Geometry check sheet. Reference: the model listing, model coordinates, mm. A direction names the side the tool comes from. Give positions to 0.01 mm unless a question says otherwise; leave off trailing zeros. Order: outer loops, then holes, each group sorted by start corner. A loop starts at its lowest first (then second) coordinate and runs counter-clockwise, first axis right, second up.
```python
from build123d import *

# Parameters (mm, degrees)
SKETCH_W     = 42
SKETCH_H     = 42
PAD_DEPTH    = 48
CHAMFER_SIZE = 4
SKETCH005_R  = 18
PAD003_DEPTH = 35
SKETCH001_R  = 11
PAD001_DEPTH = 2
SKETCH002_R  = 4
PAD002_DEPTH = 20
POCKET_DEPTH = 15
SKETCH004_R  = 1.25
HOLE_DEPTH   = 4.5
HOLE_TIPS_R  = 1.25


with BuildPart() as part:
    # Sketch → Pad (new body)
    with BuildSketch(Plane.XY):
        Rectangle(SKETCH_W, SKETCH_H)
    extrude(amount=PAD_DEPTH)

    # Chamfer
    chamfer_edges = [part.edges().sort_by_distance(p)[0] for p in [
        (21, -21, 24),
        (-21, -21, 24),
        (21, 21, 24),
        (-21, 21, 24),
    ]]
    chamfer(chamfer_edges, length=CHAMFER_SIZE)

    # Sketch005 → Pad003 (join)
    with BuildSketch(Plane.XY):
        Circle(SKETCH005_R)
    extrude(amount=-PAD003_DEPTH)

    # Sketch001 → Pad001 (join)
    with BuildSketch(Plane.XY.offset(-35)):
        Circle(SKETCH001_R)
    extrude(amount=-PAD001_DEPTH)

    # Sketch002 (on Sketch) → Pad002 (join)
    with BuildSketch(Plane.XY.offset(-35)):
        Circle(SKETCH002_R)
    extrude(amount=-PAD002_DEPTH)

    # Sketch003 (on Sketch) → Pocket (cut)
    with BuildSketch(Plane.XY.offset(-40)):
        with BuildLine():
            ThreePointArc((10.583005, 3), (0, 11), (-10.583005, 3))
            Line((-10.583005, 3), (10.583005, 3))
        make_face()
    extrude(amount=-POCKET_DEPTH, mode=Mode.SUBTRACT)

    # Sketch004 (on Sketch) → Hole (cut)
    with BuildSketch(Plane.XY.offset(-35)):
        with Locations((9.899495, 9.899495)):
            Circle(SKETCH004_R)
        with Locations((-9.899495, 9.899495)):
            Circle(SKETCH004_R)
        with Locations((-9.899495, -9.899495)):
            Circle(SKETCH004_R)
        with Locations((9.899495, -9.899495)):
            Circle(SKETCH004_R)
    extrude(amount=HOLE_DEPTH, mode=Mode.SUBTRACT)

    # Hole tips → Hole tip 1 section 0
    with BuildSketch(Plane.XY.offset(-30.5), mode=Mode.PRIVATE) as hole_tip_1_s0:
        with Locations((9.899495, 9.899495)):
            Circle(HOLE_TIPS_R)
    loft([hole_tip_1_s0.sketch, Vertex(9.899495, 9.899495, -29.748924)], mode=Mode.SUBTRACT)

    # Hole tips → Hole tip 2 section 0
    with BuildSketch(Plane.XY.offset(-30.5), mode=Mode.PRIVATE) as hole_tip_2_s0:
        with Locations((-9.899495, 9.899495)):
            Circle(HOLE_TIPS_R)
    loft([hole_tip_2_s0.sketch, Vertex(-9.899495, 9.899495, -29.748924)], mode=Mode.SUBTRACT)

    # Hole tips → Hole tip 3 section 0
    with BuildSketch(Plane.XY.offset(-30.5), mode=Mode.PRIVATE) as hole_tip_3_s0:
        with Locations((-9.899495, -9.899495)):
            Circle(HOLE_TIPS_R)
    loft([hole_tip_3_s0.sketch, Vertex(-9.899495, -9.899495, -29.748924)], mode=Mode.SUBTRACT)

    # Hole tips → Hole tip 4 section 0
    with BuildSketch(Plane.XY.offset(-30.5), mode=Mode.PRIVATE) as hole_tip_4_s0:
        with Locations((9.899495, -9.899495)):
            Circle(HOLE_TIPS_R)
    loft([hole_tip_4_s0.sketch, Vertex(9.899495, -9.899495, -29.748924)], mode=Mode.SUBTRACT)


solid = part.part
```
Q1. Thickness scan on L1, parallel to Z at x = -2, y = 7.5; L2, parallel to Z at x = 14, y = -14; L3, parallel to X at y = 7, z = -0.5. Record the ranges inside material, lowest first.
Q2. Access from +Z, -Z, +X, -X, +Y, -Y to the whole of each face (thin tool, end or side, straight path). Record for faces 1 (the face through (21, 0, 24)), 2 (the face through (0, 3, -47)), 3 (the face through (-8, -8, -35)).
Q3. Cross-section at A-A, the plane z = 21. Record the boundary of the cut face in (x, y), and give its area (3 significant figures).
Q4. Gauge pin test, flat ends, axial feed: P1, Ø12.5, axis at x = 4.5, y = 9.5, coming from the -Z side; P2, Ø2, axis at y = 6.5, z = -31.5, coming from the +X side; P3, Ø0.8, axis at x = 0, y = 3.5, coming from the -Z side. Record the tip position at first contact, or that the pin passes through.
Q5. Cross-section at D-D, the plane y = 0. Record the boundary of the cut face in (x, z).
Q6. Cross-section at C-C, the plane y = -13. Record the boundary of the cut face in (x, z).
Q7. Cross-section at B-B, the plane x = 0. Record the boundary of the cut face in (y, z), and give its area (3 significant figures).
Answers follow:
1. L1: z = -37 to 48
1. L2: z = 0 to 48
1. L3: x = -16.58 to 16.58
2. face 1: +Z, -Z, +X, +Y, -Y
2. face 2: -Z, +X, -X, +Y
2. face 3: -Z
3. outline: (-21, -17) - (-17, -21) - (17, -21) - (21, -17) - (21, 17) - (17, 21) - (-17, 21) - (-21, 17) - close
3. area: 1,730 mm2
4. P1: stops at z = -37
4. P2: stops at x = 17.14
4. P3: stops at z = -40
5. outline: (-21, 0) - (-18, 0) - (-18, -35) - (-11, -35) - (-11, -37) - (-4, -37) - (-4, -55) - (4, -55) - (4, -37) - (11, -37) - (11, -35) - (18, -35) - (18, 0) - (21, 0) - (21, 48) - (-21, 48) - close
6. outline: (-21, 0) - (-12.45, 0) - (-12.45, -35) - (12.45, -35) - (12.45, 0) - (21, 0) - (21, 48) - (-21, 48) - close
7. outline: (-21, 0) - (-18, 0) - (-18, -35) - (-11, -35) - (-11, -37) - (-4, -37) - (-4, -55) - (3, -55) - (3, -40) - (4, -40) - (4, -37) - (11, -37) - (11, -35) - (18, -35) - (18, 0) - (21, 0) - (21, 48) - (-21, 48) - close
7. area: 3,450 mm2
